Answer from the drawing. Dimensions are ordinates in mm from the lowest x, y and z of the part. Round coordinates to 2 decimals unless told otherwise and drop trailing zeros. Write each loop counter-clockwise with the first axis right and the second up, starting at its lowest first coordinate (ties: lowest second). Pieces come first, ordered by that corner, then holes. Notation, with made-up numbers: (-25.5, -27) - (29.5, -27) arc R25 ccw to (29.5, -11) - close; hole circle Ø4 at (-35, 21). An arc over 180 degrees is marked (long way). Use a Markdown table: item, result. Add a question column.
1) Find the intervals of material crossed by probe 1 along Y at (x, z) = (127, 32); probe 2 along Z at (x, y) = (29, 229); probe 3 along Y at (x, z) = (138, 56), in increasing order. Write a range as from..to.
2) A cutting plane is placed at D-D (x = 239). Give the vertices of the cut face in (y, z).
3) A cutting plane is placed at B-B (y = 127). Give the vertices of the cut face in (x, z), then the cut area to 3 significant figures.
4) Determine the mould class of the marked faces 1, 2, 3 and 4 for opening direction X: +X half, -X half, draft (parallel to the pull), parting line (faces both ways), or undercut.
5) This flat-tipped pin is pushed along its axis until it touches: P1, Ø4, axis at x = 82.5, z = 49, coming from the -Y side. Where does it stop, or does it pass through?
6) A cutting plane is placed at A-A (x = 127). Give the vertices of the cut face in (y, z), then the cut area to 3 significant figures.
7) A cutting plane is placed at C-C (z = 32). Give the vertices of the cut face in (x, y).
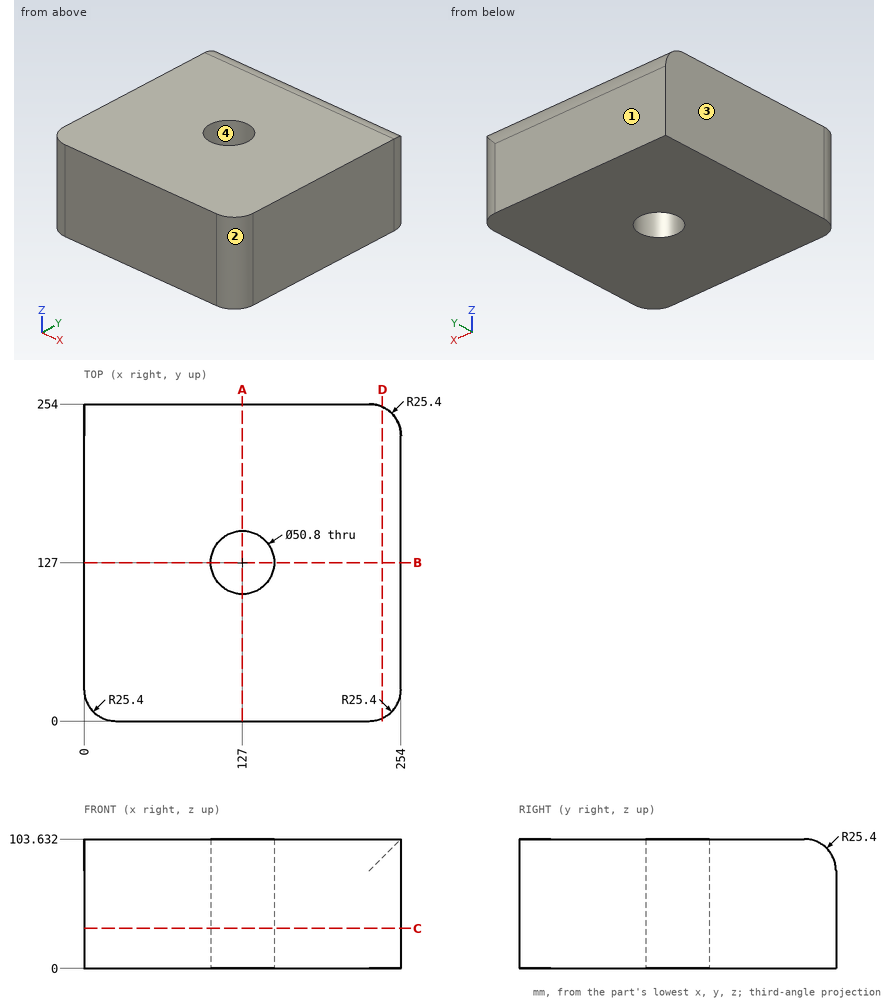
Entries:
| question | item | result |
|---|---|---|
| 1 | probe 1 | y = 0..101.6, 152.4..254 |
| 1 | probe 2 | z = 0..103.63 |
| 1 | probe 3 | y = 0..104.11, 149.89..254 |
| 2 | outline | (2.23, 0) - (251.77, 0) - (251.77, 88.63) arc R25.4 ccw to (228.6, 103.63) - (2.23, 103.63) - close |
| 3 | outline | (0, 0) - (101.6, 0) - (101.6, 103.63) - (0, 103.63) - close; (152.4, 0) - (254, 0) - (254, 103.63) - (152.4, 103.63) - close |
| 3 | area | 21,100 mm² |
| 4 | face 1 | draft |
| 4 | face 2 | +X half |
| 4 | face 3 | -X half |
| 4 | face 4 | undercut |
| 5 | P1 | stops at y = 0 |
| 6 | outline | (0, 0) - (101.6, 0) - (101.6, 103.63) - (0, 103.63) - close; (152.4, 0) - (254, 0) - (254, 78.23) arc R25.4 ccw to (228.6, 103.63) - (152.4, 103.63) - close |
| 6 | area | 20,900 mm² |
| 7 | outline | (0, 25.4) arc R25.4 ccw to (25.4, 0) - (228.6, 0) arc R25.4 ccw to (254, 25.4) - (254, 228.6) arc R25.4 ccw to (228.6, 254) - (0, 254) - close; hole circle Ø50.8 at (127, 127) |
